The listing builds one solid part. Answer for the finished solid, in the listing's coordinates (mm). A direction names the side the tool comes from. Give positions to 0.01 mm unless a question says otherwise; leave off trailing zeros. Write each loop counter-clockwise with the first axis right and the second up, starting at its lowest first coordinate (ties: lowest second). Pieces come first, ordered by that corner, then holes.
```python
from build123d import *

# Parameters (mm, degrees)
SKETCH1_W           = 9
SKETCH1_H           = 21.333333333
SKETCH1_H_2         = 21.333333334
BOSS_EXTRUDE1_DEPTH = 2
BOSS_EXTRUDE2_DEPTH = 3.59
BOSS_EXTRUDE3_DEPTH = 4


with BuildPart() as part:
    # Sketch1 → Boss-Extrude1 (new body)
    with BuildSketch(Plane.XY):
        Polygon((0, 76), (0, 0), (45, 0), (45, 12.825), (24.825, 12.825), (24.825, 63.175), (75.175, 63.175), (75.175, 12.825), (55, 12.825), (55, 0), (100, 0), (100, 76), align=None)
        with Locations((92.5, 13.666666667)):
            Rectangle(SKETCH1_W, SKETCH1_H, mode=Mode.SUBTRACT)
        with Locations((92.5, 38)):
            Rectangle(SKETCH1_W, SKETCH1_H_2, mode=Mode.SUBTRACT)
        with Locations((92.5, 62.333333334)):
            Rectangle(SKETCH1_W, SKETCH1_H, mode=Mode.SUBTRACT)
        with Locations((7.5, 62.333333334)):
            Rectangle(SKETCH1_W, SKETCH1_H, mode=Mode.SUBTRACT)
        with Locations((7.5, 38)):
            Rectangle(SKETCH1_W, SKETCH1_H_2, mode=Mode.SUBTRACT)
        with Locations((7.5, 13.666666667)):
            Rectangle(SKETCH1_W, SKETCH1_H, mode=Mode.SUBTRACT)
    extrude(amount=BOSS_EXTRUDE1_DEPTH)

    # Sketch1<3> → Boss-Extrude2 (add)
    with BuildSketch(Plane.XY):
        Polygon((15, 3), (45, 3), (45, 9.825), (21.825, 9.825), (21.825, 66.175), (78.175, 66.175), (78.175, 9.825), (55, 9.825), (55, 3), (85, 3), (85, 73), (15, 73), align=None)
    extrude(amount=BOSS_EXTRUDE2_DEPTH)

    # Sketch1<4> → Boss-Extrude3 (add)
    with BuildSketch(Plane.XY):
        Polygon((12, 3), (12, 0), (45, 0), (45, 3), (15, 3), (15, 73), (85, 73), (85, 3), (55, 3), (55, 0), (88, 0), (88, 3), (88, 24.333333333), (88, 27.333333333), (88, 48.666666667), (88, 51.666666667), (88, 73), (88, 76), (12, 76), (12, 73), (12, 51.666666667), (12, 48.666666667), (12, 27.333333333), (12, 24.333333333), align=None)
    extrude(amount=BOSS_EXTRUDE3_DEPTH)


solid = part.part
```
Item 1: Consider probe 1 along X at (y, z) = (72, 0.45); probe 2 along Y at (x, z) = (89, 0.9); probe 3 along Y at (x, z) = (42.5, 3.05) (3 decimals). Determine where each line is inside the solid, lowest interval first.
Conclusion:
probe 1: x = 0 to 3, 12 to 88, 97 to 100
probe 2: y = 0 to 3, 24.33 to 27.33, 48.67 to 51.67, 73 to 76
probe 3: y = 0 to 9.825, 66.175 to 76
Item 2: Determine the mould class of faces 1 (the face through (49, 64, 0)), 2 (the face through (24.825, 38, 1)) for opening direction Y: pulls with the +Y half, pulls with the -Y half, needs draft (parallel to the pull), parting line crosses it, or undercut.
Conclusion:
face 1: needs draft
face 2: undercut
Item 3: A cutting plane is placed at A-A, the plane y = 65. Give the vertices of the cut face in (x, z) (3 decimals), plus the area to 3 significant figures.
Conclusion:
outline: (0, 0) - (3, 0) - (3, 2) - (0, 2) - close; (12, 0) - (88, 0) - (88, 4) - (85, 4) - (85, 3.59) - (78.175, 3.59) - (78.175, 2) - (21.825, 2) - (21.825, 3.59) - (15, 3.59) - (15, 4) - (12, 4) - close; (97, 0) - (100, 0) - (100, 2) - (97, 2) - close
area: 198 mm2
Item 4: A cutting plane is placed at C-C, the plane y = 18. Give the vertices of the cut face in (x, z) (3 decimals).
Conclusion:
outline: (0, 0) - (3, 0) - (3, 2) - (0, 2) - close; (12, 0) - (24.825, 0) - (24.825, 2) - (21.825, 2) - (21.825, 3.59) - (15, 3.59) - (15, 4) - (12, 4) - close; (75.175, 0) - (88, 0) - (88, 4) - (85, 4) - (85, 3.59) - (78.175, 3.59) - (78.175, 2) - (75.175, 2) - close; (97, 0) - (100, 0) - (100, 2) - (97, 2) - close
Item 5: A cutting plane is placed at B-B, the plane x = 41.5. Give the vertices of the cut face in (y, z) (3 decimals), plus the area to 3 significant figures.
Conclusion:
outline: (0, 0) - (12.825, 0) - (12.825, 2) - (9.825, 2) - (9.825, 3.59) - (3, 3.59) - (3, 4) - (0, 4) - close; (63.175, 0) - (76, 0) - (76, 4) - (73, 4) - (73, 3.59) - (66.175, 3.59) - (66.175, 2) - (63.175, 2) - close
area: 85.0 mm2
Item 6: Each of these flat-tipped pins is pushed along its axis until it touches: P1, Ø10, axis at x = 52.5, y = 11, coming from the +Z side; P2, Ø9.5, axis at x = 6.5, y = 41.5, coming from the +Z side; P3, Ø0.5, axis at y = 27.5, z = 4, coming from the -X side. Where does it stop, or does it pass through?
Conclusion:
P1: stops at z = 3.59
P2: stops at z = 2
P3: stops at x = 12
Item 7: Which of the six approach directions +Z, -Z, +X, -X, +Y, -Y give full straight-line access (tool end or side, diameter ignored) to faces 3 (the face through (3, 62, 1)), 4 (the face through (50, 75, 4)), 5 (the face through (55, 7, 2))?
Conclusion:
face 3: +Z, -Z
face 4: +Z, +X, -X, +Y, -Y
face 5: +Z, -Z, -Y
Item 8: A cutting plane is placed at D-D, the plane x = 92.5. Give the vertices of the cut face in (y, z), plus the area to 3 significant figures.
Conclusion:
outline: (0, 0) - (3, 0) - (3, 2) - (0, 2) - close; (24.33, 0) - (27.33, 0) - (27.33, 2) - (24.33, 2) - close; (48.67, 0) - (51.67, 0) - (51.67, 2) - (48.67, 2) - close; (73, 0) - (76, 0) - (76, 2) - (73, 2) - close
area: 24.0 mm2
